For this review, take the finished solid that the model builds, in its own axes (mm). A direction names the side the tool comes from. Coordinates: 2 decimals unless noted, no trailing zeros. Write each loop counter-clockwise with the first axis right and the second up, starting at its lowest first coordinate (ties: lowest second). Pieces come first, ordered by that corner, then holes. Notation, with made-up numbers: M -3.5,17.5 L 39.5,17.5 A25 cw 39.5,29.5 Z; hole C 47,21.5 d5. An arc over 180 degrees is marked long. Return JSON: item names as keys, results as strings.
```python
from build123d import *

# Parameters (mm, degrees)
F0_R     = 4
F1_DEPTH = 34.5
F3_SIZE  = 0.1
F2_W     = 3
F2_H     = 1.5
F4_DEPTH = 15
F5_R     = 16.5
F6_DEPTH = 4
F7_R     = 1
F8_DEPTH = 4


with BuildPart() as f1:
    # F0 (on Front) → F1 (new body)
    with BuildSketch(Plane.XZ):
        Circle(F0_R)
    extrude(amount=-F1_DEPTH)

    # F3
    f3_edges = [f1.edges().sort_by_distance(p)[0] for p in [
        (-4, 0, 0),
    ]]
    chamfer(f3_edges, length=F3_SIZE)

    # F2 (on Front) → F4 (cut)
    with BuildSketch(Plane.XZ):
        with Locations((0, 3.25)):
            Rectangle(F2_W, F2_H)
    extrude(amount=-F4_DEPTH, mode=Mode.SUBTRACT)

    # F5 (on face) → F6 (join)
    with BuildSketch(Plane(origin=(0, 34.5, 0), x_dir=(-1, 0, 0), z_dir=(0, 1, 0))):
        Circle(F5_R)
    extrude(amount=F6_DEPTH)

    # F7 (on face) → F8 (join)
    with BuildSketch(Plane(origin=(0, 38.5, 0), x_dir=(-1, 0, 0), z_dir=(0, 1, 0))):
        with Locations((-0.185544, 13)):
            Circle(F7_R)
        with Locations((-13, -0.185544)):
            Circle(F7_R)
        with Locations((0.185544, -13)):
            Circle(F7_R)
        with Locations((13, 0.185544)):
            Circle(F7_R)
    extrude(amount=F8_DEPTH)


solid = f1.part
```
1. Wall thickness on L1, parallel to Y at x = -1.5, z = 9; L2, parallel to Z at x = 3, y = 4.5; L3, parallel to Z at x = 4, y = 35: over which ranges is each line inside the solid? List them lowest first. Write a range as from..to.
Checks:
{"L1": "34.5..38.5", "L2": "-2.65..2.65", "L3": "-16.01..16.01"}
2. Draft analysis for pull direction Z (two halves, no side actions). For faces 1 (the face through (-0.867, 17.059, -3.905)), 2 (the face through (0.402, 40.472, 12.024)), 3 (the face through (0, 15, 3)), state which applies: +Z half, -Z half, draft (parallel to the pull), parting line (faces both ways), or undercut.
Checks:
{"face 1": "parting line", "face 2": "undercut", "face 3": "draft"}
3. We need section B-B (y = 18.5). State the section outline as (x, z) points.
Checks:
{"outline": "C 0,0 d8"}
4. We need section C-C (x = 0). State the section outline as (y, z) points.
Checks:
{"outline": "M 0,-3.9 L 0.1,-4 L 34.5,-4 L 34.5,-16.5 L 38.5,-16.5 L 38.5,-13.98 L 42.5,-13.98 L 42.5,-12.02 L 38.5,-12.02 L 38.5,12.02 L 42.5,12.02 L 42.5,13.98 L 38.5,13.98 L 38.5,16.5 L 34.5,16.5 L 34.5,4 L 15,4 L 15,2.5 L 0,2.5 Z"}
5. We need section D-D (x = 13). State the section outline as (y, z) points, plus the area to 3 significant figures.
Checks:
{"outline": "M 34.5,-10.16 L 38.5,-10.16 L 38.5,-1.19 L 42.5,-1.19 L 42.5,0.81 L 38.5,0.81 L 38.5,10.16 L 34.5,10.16 Z", "area": "89.3 mm2"}
6. We need section A-A (z = 13). State the section outline as (x, y) points, plus the area to 3 significant figures.
Checks:
{"outline": "M -10.16,34.5 L 10.16,34.5 L 10.16,38.5 L 1.19,38.5 L 1.19,42.5 L -0.81,42.5 L -0.81,38.5 L -10.16,38.5 Z", "area": "89.3 mm2"}
7. Clearance check with flat-ended pins moving along their axes: pin 1 Ø16.5 at (x, z) = (2, -5.5) entering from -Y; pin 2 Ø12 at (y, z) = (23, -9.5) entering from +X; pin 3 Ø0.9 at (x, y) = (0.5, 6.5) entering from +Z; pin 4 Ø3 at (x, z) = (5, -4.5) entering from +Y. State where each tip first meets the part, or that it passes through.
Checks:
{"pin 1": "y = 0", "pin 2": "x = 1.94", "pin 3": "z = 2.5", "pin 4": "y = 38.5"}
8. For faces 4 (the face through (-3, 34.5, -3)), 5 (the face through (0, 7, 2.5)), 6 (the face through (-15.24, 36.47, -6.32)), 7 (the face through (0, 38.5, 0)), list the 3-axis set-ups (+Z, -Z, +X, -X, +Y, -Y) from which the entire face can be reached by the end or side of a thin tool; tool diameter is ignored.
Checks:
{"face 4": "-Y", "face 5": "+Z, -Y", "face 6": "+Y, -Y", "face 7": "+Y"}
